Answer from the drawing. Dimensions are ordinates in mm from the lowest x, y and z of the part. A direction names the side the tool comes from. Round coordinates to 2 decimals unless told otherwise and drop trailing zeros. Loops run counter-clockwise (first coordinate to the right, second up) from the corner with the lowest first, then second, coordinate; pieces in that order, holes last. Notation, with made-up numbers: (31, 74) - (49, 74) arc R23 cw to (49, 103) - close; hole circle Ø8 at (3.5, 87.5). An arc over 180 degrees is marked (long way). One line per question, with ' | ' between items. Start each with the question number.
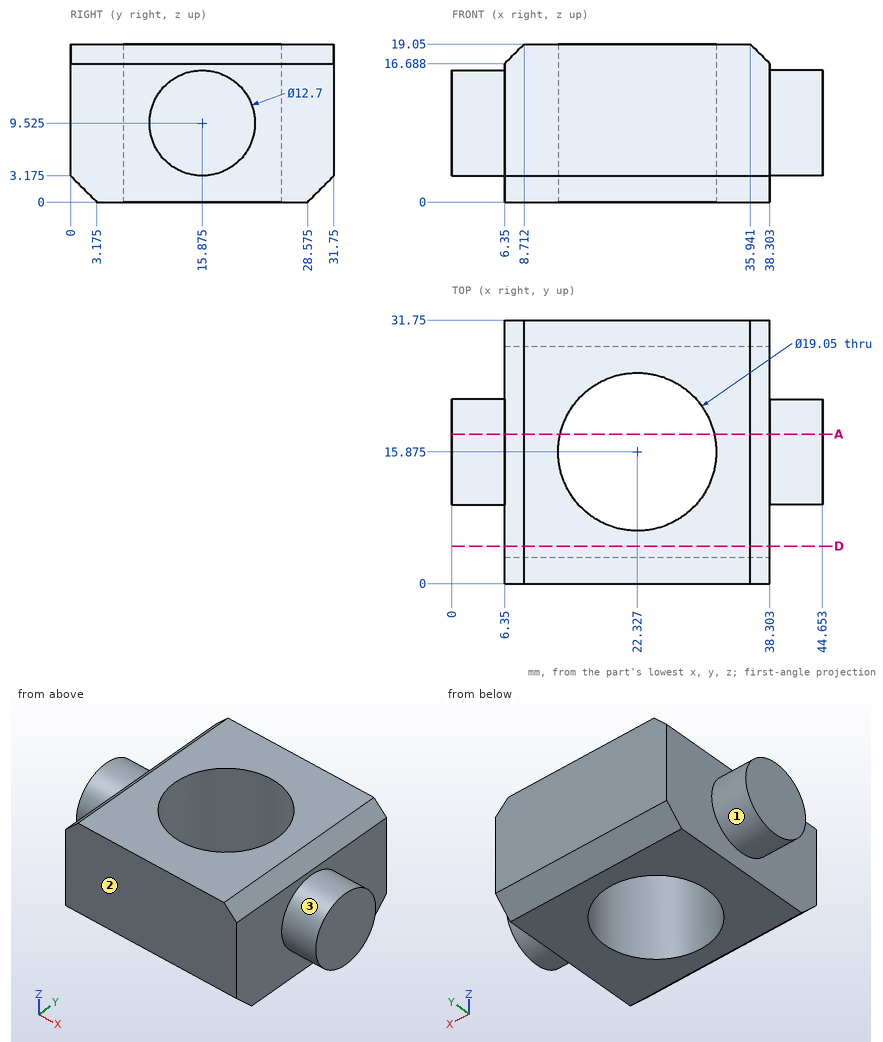
(1) Find section A-A on y = 18. Write down the section's boundary in (x, z).
(2) Each of these flat-tipped pins is pushed along its axis until it touches: P1, Ø4, axis at y = 24, z = 2, coming from the -X side; P2, Ø11.5, axis at x = 22.33, y = 15.88, coming from the +Z side; P3, Ø8, axis at y = 27, z = 11.5, coming from the +X side. Where does it stop, or does it pass through?
(3) A tool of negligible diameter and unlimited length cuts with its end or side. For the marked faces 1, 2 and 3, from which of +Z, -Z, +X, -X, +Y, -Y can it reach the whole face along a straight path? Write none if from no direction.
(4) Find section D-D on y = 4.5. Write down the section's boundary in (x, z), plus the area to 3 significant figures.
(5) Consider L1, parallel to X at y = 28, z = 1; L2, parallel to X at y = 12, z = 12.5 (1 decimal); L3, parallel to X at y = 11, z = 10.75 (1 decimal). Determine where each line is inside the solid, lowest interval first.
Answer below:
1) outline: (0, 3.54) - (6.35, 3.54) - (6.35, 0) - (13.04, 0) - (13.04, 19.05) - (8.71, 19.05) - (6.35, 16.69) - (6.35, 15.51) - (0, 15.51) - close; (31.61, 0) - (38.3, 0) - (38.3, 3.54) - (44.65, 3.54) - (44.65, 15.51) - (38.3, 15.51) - (38.3, 16.69) - (35.94, 19.05) - (31.61, 19.05) - close
2) P1: x = 6.35 | P2: through | P3: x = 38.3
3) face 1: -X | face 2: +Z, -Z, +X, -X, -Y | face 3: +X
4) outline: (6.35, 0) - (38.3, 0) - (38.3, 16.69) - (35.94, 19.05) - (8.71, 19.05) - (6.35, 16.69) - close | area: 603 mm2
5) L1: 6.35 to 38.3 | L2: 0 to 13.6, 31 to 44.7 | L3: 0 to 14.1, 30.5 to 44.7
